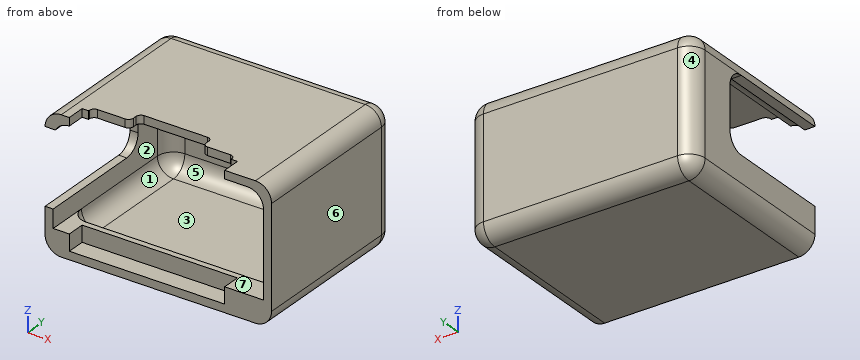
```python
from build123d import *

# Parameters (mm, degrees)
SKETCH1_W           = 140
SKETCH1_H           = 82.5
SKETCH1_W_2         = 130
SKETCH1_H_2         = 72.5
BOSS_EXTRUDE1_DEPTH = 102
BOSS_EXTRUDE2_START = 102
SKETCH1_3_W         = 140
SKETCH1_3_H         = 82.5
BOSS_EXTRUDE2_DEPTH = 5
SKETCH1_4_W         = 96
SKETCH1_4_H         = 82.405729741
BOSS_EXTRUDE4_DEPTH = 11.3
SKETCH1_5_W         = 130
SKETCH1_5_H         = 10
EXTRUDE_THIN3_DEPTH = 15
CUT_EXTRUDE2_REACH  = 157.513
SKETCH2_W           = 88
SKETCH2_H           = 15
FILLET1_R           = 10
FILLET2_R           = 10
CUT_EXTRUDE3_REACH  = 186.296
SKETCH3_W           = 46.25
SKETCH3_H           = 75
FILLET3_R           = 10
CUT_EXTRUDE4_REACH  = 157.513
SKETCH4_W           = 45
SKETCH4_H           = 12
FILLET4_R           = 3


with BuildPart() as part:
    # Sketch1 → Boss-Extrude1 (new body)
    with BuildSketch(Plane(origin=(0, 0, 0), x_dir=(1, 0, 0), z_dir=(0, 1, 0))):
        with Locations((7, 12.75)):
            Rectangle(SKETCH1_W, SKETCH1_H)
        with Locations((7, 12.75)):
            Rectangle(SKETCH1_W_2, SKETCH1_H_2, mode=Mode.SUBTRACT)
    extrude(amount=BOSS_EXTRUDE1_DEPTH)

    # Sketch1<3> → Boss-Extrude2 (add)
    with BuildSketch(Plane(origin=(0, 0, 0), x_dir=(1, 0, 0), z_dir=(0, 1, 0)).offset(BOSS_EXTRUDE2_START)):
        with Locations((7, 12.75)):
            Rectangle(SKETCH1_3_W, SKETCH1_3_H)
    extrude(amount=BOSS_EXTRUDE2_DEPTH)

    # Sketch1<5> → Extrude-Thin3 (add)
    with BuildSketch(Plane(origin=(0, 0, 0), x_dir=(1, 0, 0), z_dir=(0, 1, 0))):
        with Locations((7, 44)):
            Rectangle(SKETCH1_5_W, SKETCH1_5_H)
    extrude(amount=EXTRUDE_THIN3_DEPTH)


with BuildPart() as body_2:
    # Sketch1<4> → Boss-Extrude4 (new body)
    with BuildSketch(Plane(origin=(0, 0, 0), x_dir=(1, 0, 0), z_dir=(0, 1, 0))):
        with Locations((0, 7.797135129)):
            Rectangle(SKETCH1_4_W, SKETCH1_4_H)
    extrude(amount=BOSS_EXTRUDE4_DEPTH)


with BuildPart() as part_1:
    add(part.part)

    # Combine1: cut body 2
    add(body_2.part, mode=Mode.SUBTRACT)

    # Sketch2 → Cut-Extrude2 (cut, up to next)
    with BuildSketch(Plane.XY.offset(28.5), mode=Mode.PRIVATE) as cut_extrude2_sk1:
        with Locations((0, 7.5)):
            Rectangle(SKETCH2_W, SKETCH2_H)
    cut_extrude2_tool1 = extrude(cut_extrude2_sk1.sketch, amount=-CUT_EXTRUDE2_REACH, mode=Mode.PRIVATE) & part_1.part
    add(cut_extrude2_tool1.solids().sort_by_distance((0, 7.5, 28.5))[0], mode=Mode.SUBTRACT)

    # Fillet1
    fillet1_edges = [part_1.edges().sort_by_distance(p)[0] for p in [
        (-58, 102, -12.75),
        (7, 102, 23.5),
        (72, 102, -12.75),
        (7, 102, -49),
        (7, 107, 28.5),
        (-63, 107, -12.75),
        (7, 107, -54),
        (77, 107, -12.75),
        (-58, 58.5, -49),
        (72, 58.5, -49),
        (72, 51, 23.5),
        (-58, 51, 23.5),
        (-63, 53.5, 28.5),
        (-63, 53.5, -54),
        (77, 53.5, -54),
        (77, 53.5, 28.5),
    ]]
    fillet(fillet1_edges, radius=FILLET1_R)

    # Fillet2
    fillet2_edges = [part_1.edges().sort_by_distance(p)[0] for p in [
        (7, 15, -49),
        (69.071067812, 15, -46.071067812),
        (-55.071067812, 15, -46.071067812),
    ]]
    fillet(fillet2_edges, radius=FILLET2_R - 0.0001)  # a hair under: the kernel refuses the full size

    # Sketch3 → Cut-Extrude3 (cut, up to next)
    with BuildSketch(Plane.ZY.offset(63), mode=Mode.PRIVATE) as cut_extrude3_sk1:
        with Locations((-4.625, 37.5)):
            Rectangle(SKETCH3_W, SKETCH3_H)
    cut_extrude3_tool1 = extrude(cut_extrude3_sk1.sketch, amount=-CUT_EXTRUDE3_REACH, mode=Mode.PRIVATE) & part_1.part
    add(cut_extrude3_tool1.solids().sort_by_distance((-63, 37.5, -4.625))[0], mode=Mode.SUBTRACT)

    # Fillet3
    fillet3_edges = [part_1.edges().sort_by_distance(p)[0] for p in [
        (-59.830127019, 75, 18.5),
        (-60.5, 75, -27.75),
    ]]
    fillet(fillet3_edges, radius=FILLET3_R)

    # Sketch4 → Cut-Extrude4 (cut, up to next)
    with BuildSketch(Plane.XY.offset(28.5), mode=Mode.PRIVATE) as cut_extrude4_sk1:
        with Locations((1.5, 17.3)):
            Rectangle(SKETCH4_W, SKETCH4_H)
    cut_extrude4_tool1 = extrude(cut_extrude4_sk1.sketch, amount=-CUT_EXTRUDE4_REACH, mode=Mode.PRIVATE) & part_1.part
    add(cut_extrude4_tool1.solids().sort_by_distance((1.5, 17.3, 28.5))[0], mode=Mode.SUBTRACT)

    # Fillet4
    fillet4_edges = [part_1.edges().sort_by_distance(p)[0] for p in [
        (44, 15, 26),
        (-44, 15, 26),
        (24, 15, 26),
        (24, 23.3, 26),
        (-21, 23.3, 26),
        (-21, 15, 26),
    ]]
    fillet(fillet4_edges, radius=FILLET4_R)


solid = part_1.part
```
Geometry: final body of the model. Coordinates: model frame, mm. Face numbers are marked on the shaded views. A direction names the side the tool comes from. Coordinates: 2 decimals unless noted, no trailing zeros. Order: outer loops, then holes, each group sorted by start corner. A loop starts at its lowest first (then second) coordinate and runs counter-clockwise, first axis right, second up.
Item 1: Draft query along Y for the marked faces 1, 2, 3 and 4. Return one class per face: released by +Y, released by -Y, zero draft, split by the parting line, or undercut.
Answer:
face 1: undercut
face 2: zero draft
face 3: undercut
face 4: released by +Y
Item 2: Section query B-B (z = -12.5). Output: boundary loops of the cut face in (x, y).
Answer:
outline: (-63, 75) - (-58, 75) - (-58, 92) arc R10 cw to (-48, 102) - (62, 102) arc R10 cw to (72, 92) - (72, 0) - (77, 0) - (77, 97) arc R10 ccw to (67, 107) - (-53, 107) arc R10 ccw to (-63, 97) - close
Item 3: Contact query for flat-ended pins moving along their axis: P1, Ø6, axis at x = -41, z = 5.5, coming from the -Y side; P2, Ø1.8, axis at y = 19.5, z = 26, coming from the +X side; P3, Ø2, axis at x = 46, z = 25.5, coming from the -Y side; P4, Ø20, axis at x = -22, y = 14, coming from the +Z side. Output: stop coordinate, or through.
Answer:
P1: stops at y = 102
P2: stops at x = 74.51
P3: stops at y = 11.3
P4: stops at z = 28.5
Item 4: Material intervals for line 1 along X through (y, z) = (76.5, -39.5); line 2 along Z through (x, y) = (-36, 39.5); line 3 along Z through (x, y) = (-27, 9.5), sorted ascending.
Answer:
line 1: x = -63 to -57.99, 71.99 to 77
line 2: z = -54 to -49, 23.5 to 28.5
line 3: z = -54 to -49
Item 5: Access query for the marked faces 5, 6 and 7. Directions: +Z, -Z, +X, -X, +Y, -Y. A direction counts if a zero-diameter tool reaches every point of the face in a straight line with its end or side. Return the directions, or none.
Answer:
face 5: none
face 6: +Z, -Z, +X, +Y, -Y
face 7: -Y
Item 6: Section query A-A (y = 62). Output: boundary loops of the cut face in (x, z).
Answer:
outline: (-63, -44) arc R10 ccw to (-53, -54) - (67, -54) arc R10 ccw to (77, -44) - (77, 18.5) arc R10 ccw to (67, 28.5) - (-53, 28.5) arc R10 ccw to (-63, 18.5) - (-56.66, 18.5) arc R10 cw to (-48, 23.5) - (62, 23.5) arc R10 cw to (72, 13.5) - (72, -39) arc R10 cw to (62, -49) - (-48, -49) arc R10 cw to (-58, -39) - (-58, -27.75) - (-63, -27.75) - close
